from build123d import *

# Parameters (mm, degrees)
F0_W = 18
F0_H = 45
F3_D = 6
F5_T = -2.5
F6_D = 89
F8_D = 2


with BuildPart() as f1:
    # F0 (on Front) → F1 (revolve)
    with BuildSketch(Plane.XZ):
        with Locations((9, 22.5)):
            Rectangle(F0_W, F0_H)
    revolve(axis=Axis((9, 0, 0), (1, 0, 0)))

    # F3 (through all)
    with Locations(Plane(origin=(0, 0, 0), x_dir=(0, 1, 0), z_dir=(-1, 0, 0))):
        with Locations((0, 0)):
            Hole(F3_D / 2)

    # F5
    f5_openings = [f1.faces().sort_by_distance(p)[0] for p in [
        (18, 0, -43.727208),
    ]]
    offset(amount=F5_T, openings=f5_openings)

    # F6 (through all)
    with Locations(Plane(origin=(0, 0, 0), x_dir=(0, 1, 0), z_dir=(-1, 0, 0))):
        with Locations((0, -21.7700034969)):
            Hole(F6_D / 2)

    # F8 (through all)
    with Locations(Plane(origin=(0, 0, 0), x_dir=(0, 1, 0), z_dir=(-1, 0, 0))):
        with Locations((-39.3494814634, 5.6586829014)):
            Hole(F8_D / 2)


solid = f1.part
The listing builds one solid part. Answer for the finished solid, in the listing's coordinates (mm). Round coordinates to 2 decimals unless told otherwise and drop trailing zeros. Order: outer loops, then holes, each group sorted by start corner. A loop starts at its lowest first (then second) coordinate and runs counter-clockwise, first axis right, second up. Notation, with made-up numbers: (49, 32) -> (62, 32) arc R29 ccw to (62, 67) -> close; hole circle Ø11 at (-30.75, -34). An arc over 180 degrees is marked (long way). One line per item, written item: value.
Item 1: Find section D-D, the plane z = 0. Give the vertices of the cut face in (x, y).
Taken from the geometry:
outline: (0, -45) -> (18, -45) -> (18, -42.5) -> (2.5, -42.5) -> (2.5, -38.81) -> (0, -38.81) -> close; (0, 38.81) -> (2.5, 38.81) -> (2.5, 42.5) -> (18, 42.5) -> (18, 45) -> (0, 45) -> close
Item 2: Find section C-C, the plane z = -30. Give the vertices of the cut face in (x, y).
Taken from the geometry:
outline: (0, -33.54) -> (18, -33.54) -> (18, -30.1) -> (2.5, -30.1) -> (2.5, 30.1) -> (18, 30.1) -> (18, 33.54) -> (0, 33.54) -> close
Item 3: Find section A-A, the plane z = -21. Give the vertices of the cut face in (x, y), then the cut area to 3 significant figures.
Taken from the geometry:
outline: (0, -39.8) -> (18, -39.8) -> (18, -36.95) -> (2.5, -36.95) -> (2.5, -12.29) -> (0, -12.29) -> close; (0, 12.29) -> (2.5, 12.29) -> (2.5, 36.95) -> (18, 36.95) -> (18, 39.8) -> (0, 39.8) -> close
area: 226 mm2
Item 4: Find section B-B, the plane y = 0. Give the vertices of the cut face in (x, z), then the cut area to 3 significant figures.
Taken from the geometry:
outline: (0, -45) -> (18, -45) -> (18, -42.5) -> (2.5, -42.5) -> (2.5, -22.73) -> (0, -22.73) -> close
area: 94.4 mm2
Item 5: For a pull along Y with two mould halves and no side action, classify faces 1 (the cylindrical face through (10.358, -1.031, -42.487)), 2 (the cylindrical face through (9.126, -1.158, -44.985)), 3 (the flat face through (18, 0, -44)) as released by +Y, released by -Y, zero draft, split by the parting line, or undercut.
Taken from the geometry:
face 1: undercut
face 2: split by the parting line
face 3: zero draft
Item 6: Given P1, Ø8, axis at x = 3.5, z = -17, coming from the -Y side; P2, Ø5, axis at x = 2.5, z = -31, coming from the +Y side; P3, Ø4, axis at x = 3, z = -38, coming from the -Y side, each flat-ended and moving along its own axis, determine where each tip first touches the part or whether it passes through.
Taken from the geometry:
P1: stops at y = -43.08
P2: stops at y = 34.82
P3: stops at y = -27
Item 7: Straight lines are drawn through the part: L1, parallel to Y at x = 13.5, z = 0; L2, parallel to X at y = 14.5, z = -39.5; L3, parallel to Y at x = 13, z = -26. For each, find the intervals that lie inside material, in ascending order.
Taken from the geometry:
L1: y = -45 to -42.5, 42.5 to 45
L2: x = 0 to 2.5
L3: y = -36.73 to -33.62, 33.62 to 36.73
